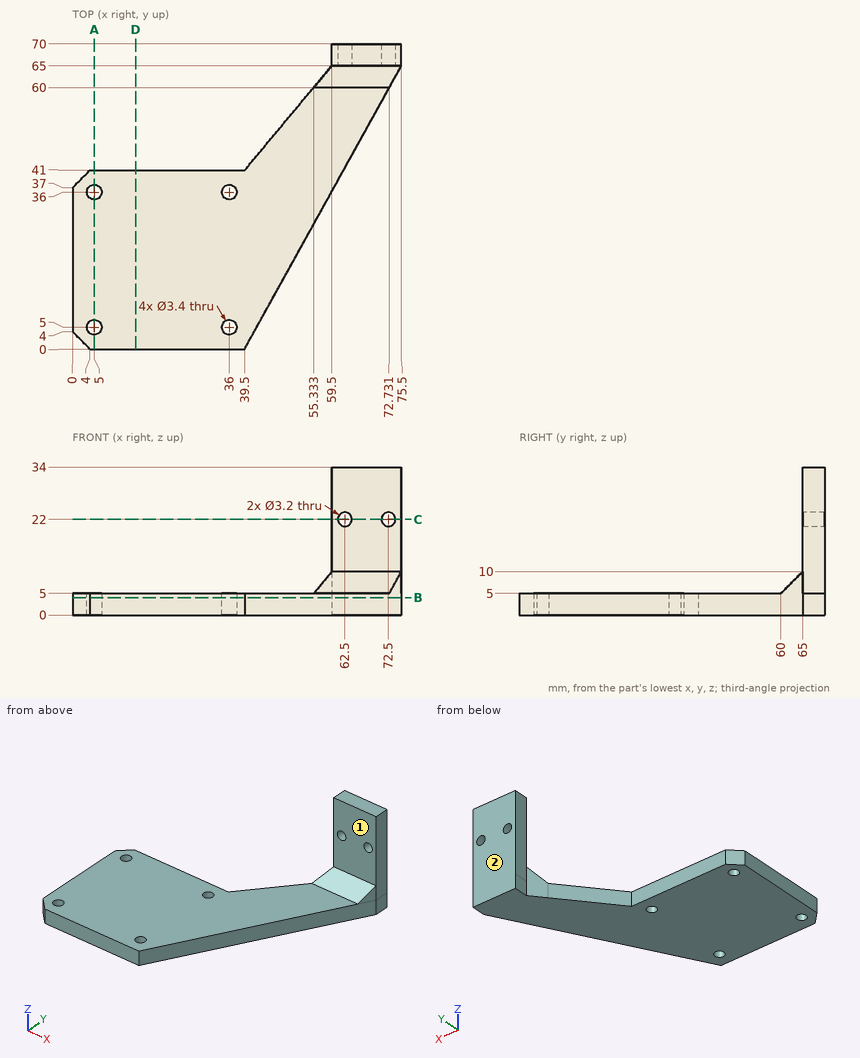
For this review, use the dimensioned drawing (mm, ordinates from the lowest corner) and the shaded views. A direction names the side the tool comes from. Round coordinates to 2 decimals unless told otherwise and drop trailing zeros. Write each loop counter-clockwise with the first axis right and the second up, starting at its lowest first coordinate (ties: lowest second). Pieces come first, ordered by that corner, then holes. Notation, with made-up numbers: (60, 26.5) - (68, 26.5) arc R26 ccw to (68, 47.5) - close; hole circle Ø8 at (33.5, -17.75). An arc over 180 degrees is marked (long way). Answer as CSV lines item,"result". Start each with the question number.
(1) We need section C-C on z = 22. State the section outline as (x, y) points, plus the area to 3 significant figures.
(2) For the marked faces 1 and 2, list the 3-axis set-ups (+Z, -Z, +X, -X, +Y, -Y) from which the entire face can be reached by the end or side of a thin tool; tool diameter is ignored.
(3) For pin 1 Ø4 at (x, y) = (5, 5) entering from +Z; pin 2 Ø17.5 at (x, z) = (65.5, 15.5) entering from -Y; pin 3 Ø1.5 at (x, z) = (13, 3.5) entering from +Y, all flat-tipped, find the tip position at first contact; note any pin that passes through.
(4) We need section A-A on x = 5. State the section outline as (y, z) points.
(5) To check wall thickness, follow line 1 (Y direction, x = 5, z = 3.55); line 2 (X direction, y = 67.2, z = 22); line 3 (Y direction, x = 23.5, z = 3.5). State the ranges of each line that lie inside material, in increasing order.
(6) We need section D-D on x = 14.5. State the section outline as (y, z) points, plus the area to 3 significant figures.
(7) We need section B-B on z = 4. State the section outline as (x, y) points.
Worked answers:
1,outline,"(59.5, 65) - (60.9, 65) - (60.9, 70) - (59.5, 70) - close; (64.1, 65) - (70.9, 65) - (70.9, 70) - (64.1, 70) - close; (74.1, 65) - (75.5, 65) - (75.5, 70) - (74.1, 70) - close"
1,area,"48.0 mm²"
2,face 1,"+Z, +X, -X, -Y"
2,face 2,"+Z, -Z, +X, -X, +Y"
3,pin 1,"z = 5"
3,pin 2,"y = 61.75"
3,pin 3,"y = 41"
4,outline,"(0, 0) - (3.3, 0) - (3.3, 5) - (0, 5) - close; (6.7, 0) - (34.3, 0) - (34.3, 5) - (6.7, 5) - close; (37.7, 0) - (41, 0) - (41, 5) - (37.7, 5) - close"
5,line 1,"0 to 3.3, 6.7 to 34.3, 37.7 to 41"
5,line 2,"59.5 to 60.9, 64.1 to 70.9, 74.1 to 75.5"
5,line 3,"0 to 41"
6,outline,"(0, 0) - (41, 0) - (41, 5) - (0, 5) - close"
6,area,"205 mm²"
7,outline,"(0, 4) - (4, 0) - (39.5, 0) - (75.5, 65) - (75.5, 70) - (59.5, 70) - (59.5, 65) - (39.5, 41) - (4, 41) - (0, 37) - close; hole circle Ø3.4 at (5, 5); hole circle Ø3.4 at (5, 36); hole circle Ø3.4 at (36, 5); hole circle Ø3.4 at (36, 36)"
